from build123d import *

# Parameters (mm, degrees)
WYTNIJ_WYCI_GNI_CIE1_DEPTH = 3
ZAOKR_GLENIE2_R            = 0.375


with BuildPart() as part:
    # Szkic1 → Obrót1 (revolve)
    with BuildSketch(Plane.XY, mode=Mode.PRIVATE) as obr_t1_sk:
        Polygon((0, 0), (0, 5.082013072), (0.53, 6), (3, 6), (3, 2.25), (3.75, 2.25), (3.75, 3), (7.8, 3), (7.8, 2), (8.8, 2.5), (14.27, 2.5), (14.8, 1.582013072), (14.8, 0), align=None)
    revolve(obr_t1_sk.sketch.rotate(Axis((0, 0, 0), (1, 0, 0)), 90), axis=Axis((0, 0, 0), (1, 0, 0)))

    # Szkic2 → Wytnij-wyciągnięcie1 (cut)
    with BuildSketch(Plane.ZY):
        Polygon((0, -1.732050808), (1.5, -0.866025404), (1.5, 0.866025404), (0, 1.732050808), (-1.5, 0.866025404), (-1.5, -0.866025404), align=None)
    extrude(amount=-WYTNIJ_WYCI_GNI_CIE1_DEPTH, mode=Mode.SUBTRACT)

    # Szkic3 → Wycięcie-obrót1 (revolve, cut)
    with BuildSketch(Plane.XY, mode=Mode.PRIVATE) as wyci_cie_obr_t1_sk:
        Polygon((3, 0), (3, 1.732050808), (3.807668556, 0), align=None)
    revolve(wyci_cie_obr_t1_sk.sketch.rotate(Axis((-0.90277096, 0, 0), (1, 0, 0)), 90), axis=Axis((-0.90277096, 0, 0), (1, 0, 0)), mode=Mode.SUBTRACT)

    # Zaokrąglenie2
    zaokr_glenie2_edges = [part.edges().sort_by_distance(p)[0] for p in [
        (7.8, 0, -2),
        (3.75, 0, -2.25),
        (3, 0, -2.25),
    ]]
    fillet(zaokr_glenie2_edges, radius=ZAOKR_GLENIE2_R - 0.0001)  # a hair under: the kernel refuses the full size


solid = part.part
Geometry check sheet. Reference: the model listing, model coordinates, mm. A direction names the side the tool comes from. Coordinates: 2 decimals unless noted, no trailing zeros. Order: outer loops, then holes, each group sorted by start corner. A loop starts at its lowest first (then second) coordinate and runs counter-clockwise, first axis right, second up. Notation, with made-up numbers: (-39.75, 70.25) -> (7.25, 70.25) arc R19 ccw to (7.25, 74.25) -> close; hole circle Ø10 at (87, 26.5). An arc over 180 degrees is marked (long way). Use a Markdown table: item, result. Add a question column.
1. Material ranges on L1, parallel to X at y = 1.75, z = -4.25; L2, parallel to Y at x = 3.25, z = -0.5; L3, parallel to Z at x = 9, y = -2.25, recorded low to high.
2. Mould release check, pull along X, two halves, no side actions. Record for faces 4 (the face through (1, 0, -1.5)), 5 (the face through (3.75, 2, -2)), 6 (the face through (14.8, 0, 0)): pulls with the +X half, pulls with the -X half, needs draft (parallel to the pull), parting line crosses it, or undercut.
3. Cross-section at A-A (x = 7.5). Enter the section's corners in (y, z), and give its area (3 significant figures).
4. Go/stop test with flat-tipped pins: pin 1 Ø0.9 at (x, y) = (1, 0.5) entering from +Z; pin 2 Ø4 at (x, z) = (13, -1) entering from +Y; pin 3 Ø4 at (x, y) = (5.5, -1) entering from +Z; pin 4 Ø5 at (y, z) = (-4, -2) entering from +X. Record where each tip stops, or that it passes through.
5. Set-up check for faces 1 (the face through (1.479, 1.293, 0.76)), 2 (the face through (5.8, -0.9, 2.86)), 3 (the face through (1.782, -1.802, 5.723)): record each of +Z, -Z, +X, -X, +Y, -Y from which the full face is reachable in a straight line by a thin tool's end or side.
Filled sheet:
| question | item | result |
|---|---|---|
| 1 | L1 | 0 to 3 |
| 1 | L2 | -2.22 to -1.09, 1.09 to 2.22 |
| 1 | L3 | -1.09 to 1.09 |
| 2 | face 4 | needs draft |
| 2 | face 5 | undercut |
| 2 | face 6 | pulls with the +X half |
| 3 | outline | circle Ø6 at (0, 0) |
| 3 | area | 28.3 mm2 |
| 4 | pin 1 | z = 6 |
| 4 | pin 2 | y = 2.5 |
| 4 | pin 3 | z = 3 |
| 4 | pin 4 | x = 14.57 |
| 5 | face 1 | -X |
| 5 | face 2 | +X |
| 5 | face 3 | +X, -X |
